from build123d import *

# Parameters (mm, degrees)
SKETCH1_W           = 50
SKETCH1_H           = 35
BOSS_EXTRUDE1_DEPTH = 8
SKETCH2_R           = 14
BOSS_EXTRUDE2_DEPTH = 25
SKETCH3_R           = 12
BOSS_EXTRUDE3_DEPTH = 43
FILLET1_R           = 5
FILLET2_R           = 1


with BuildPart() as part:
    # Sketch1 → Boss-Extrude1 (new body)
    with BuildSketch(Plane(origin=(0, 0, 0), x_dir=(1, 0, 0), z_dir=(0, 1, 0))):
        Rectangle(SKETCH1_W, SKETCH1_H)
    extrude(amount=BOSS_EXTRUDE1_DEPTH)

    # Sketch2 → Boss-Extrude2 (add)
    with BuildSketch(Plane(origin=(0, 8, 0), x_dir=(1, 0, 0), z_dir=(0, 1, 0))):
        with Locations(Location((-7, 0, 0), (0, 0, 270))):
            Circle(SKETCH2_R)
    extrude(amount=BOSS_EXTRUDE2_DEPTH)

    # Sketch3 → Boss-Extrude3 (add)
    with BuildSketch(Plane(origin=(0, 33, 0), x_dir=(1, 0, 0), z_dir=(0, 1, 0))):
        with Locations(Location((-7, 0, 0), (0, 0, 270))):
            Circle(SKETCH3_R)
    extrude(amount=BOSS_EXTRUDE3_DEPTH)

    # Fillet1
    fillet1_edges = [part.edges().sort_by_distance(p)[0] for p in [
        (25, 4, 17.5),
        (-25, 4, 17.5),
        (-25, 4, -17.5),
        (25, 4, -17.5),
    ]]
    fillet(fillet1_edges, radius=FILLET1_R)

    # Fillet2
    fillet2_edges = [part.edges().sort_by_distance(p)[0] for p in [
        (-7, 33, -14),
        (-7, 76, -12),
    ]]
    fillet(fillet2_edges, radius=FILLET2_R)


solid = part.part
Read the model definition and answer for the solid it produces. Units are mm, in the model's axes. A direction names the side the tool comes from. Round coordinates to 2 decimals unless told otherwise and drop trailing zeros. Order: outer loops, then holes, each group sorted by start corner. A loop starts at its lowest first (then second) coordinate and runs counter-clockwise, first axis right, second up.
1) Flat-ended cylindrical pins translate along their axes: pin 1 (2 mm diameter, centred on y = 44.5, z = -6, fed in from +X); pin 2 (10 mm diameter, centred on x = 11.5, z = -8.5, fed in from +Y); pin 3 (4 mm diameter, centred on y = 41.5, z = -9, fed in from -X); pin 4 (12 mm diameter, centred on x = 16.5, y = 24.5, fed in from +Z). Find the tip coordinate at first contact, or state that the pin passes through.
2) Straight lines are drawn through the part: L1, parallel to Y at x = 6.5, z = -6.5; L2, parallel to Y at x = -13.5, z = -9; L3, parallel to X at y = 67, z = 9. For each, find the intervals that lie inside material, in ascending order.
3) The part is cut by section C-C on y = 40.5. Write down the section's boundary in (x, z).
4) The part is cut by section D-D on x = 8. Write down the section's boundary in (y, z).
5) The part is cut by section B-B on x = -7. Write down the section's boundary in (y, z).
6) The part is cut by section A-A on z = 0. Write down the section's boundary in (x, y), plus the area to 3 significant figures.
7) For faces 1 (the face through (-16, 33, 9)), 2 (the face through (0, 0, 0)), determine the directions among +Z, -Z, +X, -X, +Y, -Y from which every point of the face is accessible in a straight line to the end or side of a thin tool.
Resolved:
1. pin 1: stops at x = 3.91
1. pin 2: stops at y = 8
1. pin 3: stops at x = -16.75
1. pin 4: passes through
2. L1: y = 0 to 8
2. L2: y = 0 to 75.99
2. L3: x = -14.94 to 0.94
3. outline: circle Ø24 at (-7, 0)
4. outline: (0, -17.5) - (8, -17.5) - (8, 17.5) - (0, 17.5) - close
5. outline: (0, -17.5) - (8, -17.5) - (8, -14) - (32, -14) arc R1 ccw to (33, -13) - (33, -12) - (75, -12) arc R1 ccw to (76, -11) - (76, 11) arc R1 ccw to (75, 12) - (33, 12) - (33, 13) arc R1 ccw to (32, 14) - (8, 14) - (8, 17.5) - (0, 17.5) - close
6. outline: (-25, 0) - (25, 0) - (25, 8) - (7, 8) - (7, 32) arc R1 ccw to (6, 33) - (5, 33) - (5, 75) arc R1 ccw to (4, 76) - (-18, 76) arc R1 ccw to (-19, 75) - (-19, 33) - (-20, 33) arc R1 ccw to (-21, 32) - (-21, 8) - (-25, 8) - close
6. area: 2,130 mm2
7. face 1: +Y
7. face 2: +Z, -Z, +X, -X, -Y
